Design review of the part built by this model. Coordinates are the model's own, in mm. Face numbers are marked on the shaded views. Round coordinates to 2 decimals unless told otherwise and drop trailing zeros. Loops run counter-clockwise (first coordinate to the right, second up) from the corner with the lowest first, then second, coordinate; pieces in that order, holes last. Notation, with made-up numbers: (44.5, 86) - (84.5, 86) arc R26 cw to (84.5, 114) - close; hole circle Ø1 at (41.25, 75.5). An arc over 180 degrees is marked (long way). Use one line per item in the form item = value. Start each with the question number.
(1) Wall thickness on probe 1 along X at (y, z) = (20.75, 82) (3 decimals); probe 2 along Y at (x, z) = (33.5, 89) (3 decimals): over which ranges is each line inside the solid? List them lowest first. Write a range as [from, to].
(2) We need section C-C, the plane z = 40. Write out the cut boundary in (x, y) (3 decimals).
(3) We need section A-A, the plane x = 25.4. Write out the cut boundary in (y, z) (1 decimal).
(4) For pin 1 (1 mm diameter, centred on x = 26.5, z = 62.5, fed in from -Y); pin 2 (13.5 mm diameter, centred on x = 32, z = 77.5, fed in from +Y) (3 decimals), all flat-tipped, find the tip position at first contact; note any pin that passes through.
(5) We need section D-D, the plane z = 167. Write out the cut boundary in (x, y) (3 decimals), then the cut area to 3 significant figures.
(6) We need section B-B, the plane y = 23.75. Write out the cut boundary in (x, z) (3 decimals), then the cut area to 3 significant figures.
(7) The part is to be moulded in two halves that separate along X. For the marked faces 1, 2, 3 and 4, say which applies: released by +X, released by -X, zero draft, split by the parting line, or undercut.
from build123d import *

# Parameters (mm, degrees)
EXTRUDE_F_DEPTH    = 192.024
CUT_EXTRUDE1_REACH = 201.869
SKETCH2_R          = 14.2875


with BuildPart() as part:
    # Sketch1 → Extrude f (new body)
    with BuildSketch(Plane.XY):
        Polygon((3.175, 3.175), (3.175, 25.4), (0, 25.4), (0, 0), (50.8, 0), (50.8, 25.4), (47.625, 25.4), (47.625, 3.175), align=None)
    extrude(amount=EXTRUDE_F_DEPTH)

    # Sketch2 → Cut-Extrude1 (cut, up to next)
    with BuildSketch(Plane(origin=(0, 3.175, 0), x_dir=(1, 0, 0), z_dir=(0, 1, 0)), mode=Mode.PRIVATE) as cut_extrude1_sk1:
        with Locations(Location((25.4, -166.624, 0), (0, 0, 270))):
            Circle(SKETCH2_R)
    cut_extrude1_tool1 = extrude(cut_extrude1_sk1.sketch, amount=-CUT_EXTRUDE1_REACH, mode=Mode.PRIVATE) & part.part
    add(cut_extrude1_tool1.solids().sort_by_distance((25.4, 3.175, 166.624))[0], mode=Mode.SUBTRACT)


solid = part.part
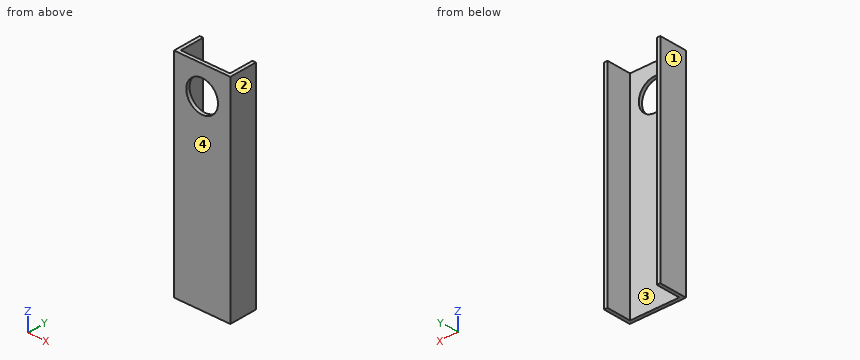
Data:
q1.probe_1 = [0, 3.175], [47.625, 50.8]
q1.probe_2 = [0, 3.175]
q2.outline = (0, 0) - (50.8, 0) - (50.8, 25.4) - (47.625, 25.4) - (47.625, 3.175) - (3.175, 3.175) - (3.175, 25.4) - (0, 25.4) - close
q3.outline = (0, 0) - (3.2, 0) - (3.2, 152.3) - (0, 152.3) - close; (0, 180.9) - (3.2, 180.9) - (3.2, 192) - (0, 192) - close
q4.pin_1 = 0
q4.pin_2 = 3.175
q5.outline = (0, 0) - (11.117, 0) - (11.117, 3.175) - (3.175, 3.175) - (3.175, 25.4) - (0, 25.4) - close; (39.683, 0) - (50.8, 0) - (50.8, 25.4) - (47.625, 25.4) - (47.625, 3.175) - (39.683, 3.175) - close
q5.area = 212 mm^2
q6.outline = (0, 0) - (3.175, 0) - (3.175, 192.024) - (0, 192.024) - close; (47.625, 0) - (50.8, 0) - (50.8, 192.024) - (47.625, 192.024) - close
q6.area = 1,220 mm^2
q7.face_1 = released by -X
q7.face_2 = released by +X
q7.face_3 = undercut
q7.face_4 = zero draft
